Design review of the part shown in the three views and the two pictorial views. Dimensions are in mm from the part's minimum x, y and z. Round coordinates to 2 decimals unless told otherwise and drop trailing zeros. Loops run counter-clockwise (first coordinate to the right, second up) from the corner with the lowest first, then second, coordinate; pieces in that order, holes last. Notation, with made-up numbers: M -38.75,18.25 L 12.25,18.25 A23 cw 12.25,42.25 Z; hole C 79.5,75.5 d9. An arc over 180 degrees is marked long. Return JSON: item names as keys, results as strings. Group by question number.
Q1. Consider section B-B (z = 30). State the section outline as (x, y) points, and give its area (3 significant figures).
Q2. Draft analysis for pull direction X (two halves, no side actions). For the marked faces 1 and 2, state which applies: pulls with the +X half, pulls with the -X half, needs draft (parallel to the pull), parting line crosses it, or undercut.
Q3. Consider section C-C (x = 10). State the section outline as (y, z) points, and give its area (3 significant figures).
Q4. To check wall thickness, follow line 1 along X through (y, z) = (3.3, 30); line 2 along X through (y, z) = (2, 30); line 3 along X through (y, z) = (3.1, 28). State the ranges of each line that lie inside material, in increasing order.
Q5. Consider section D-D (z = 24). State the section outline as (x, y) points, and give its area (3 significant figures).
Q6. Consider section A-A (x = 30). State the section outline as (y, z) points, and give its area (3 significant figures).
Q7. Clearance check with flat-ended pins moving along their axes: pin 1 Ø3.5 at (x, z) = (30, 30) entering from +Y; pin 2 Ø1.7 at (y, z) = (2.5, 30) entering from +X; pin 3 Ø2 at (x, y) = (17.5, 2.5) entering from -Z; pin 4 Ø5 at (x, z) = (8, 29) entering from +Y. State where each tip first meets the part, or that it passes through.
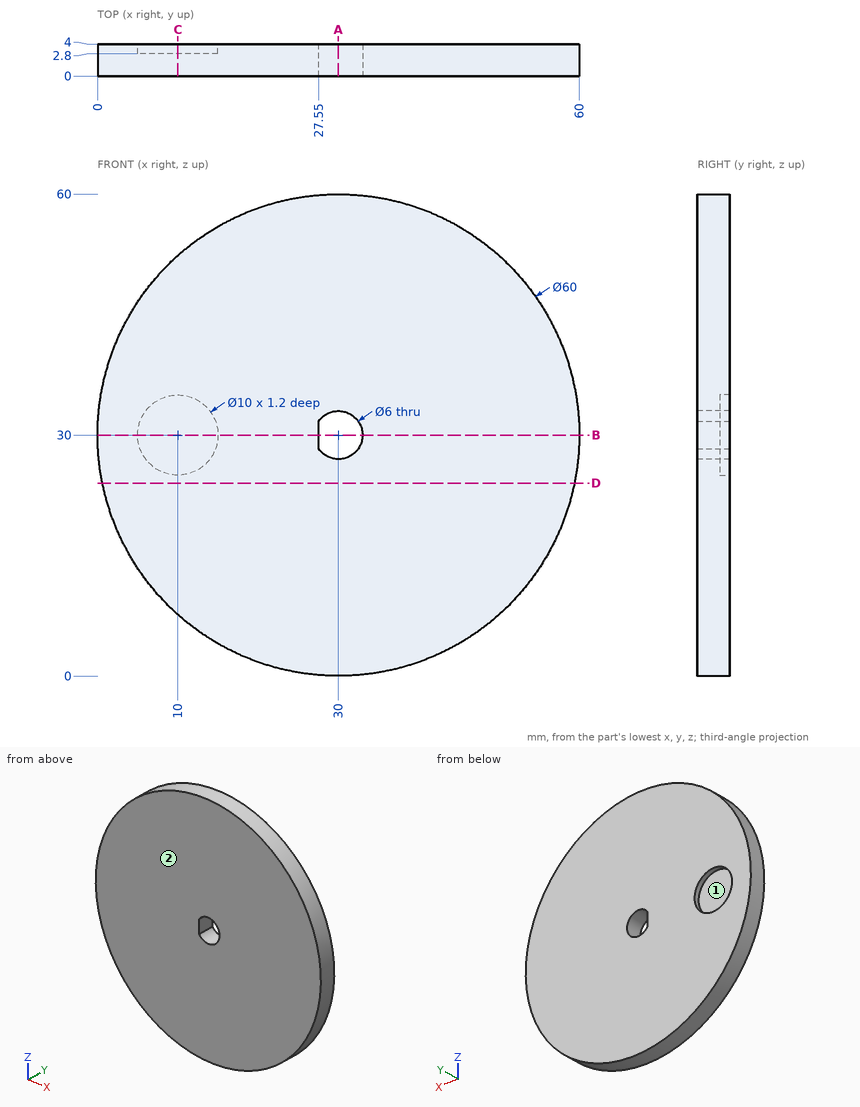
Values:
{
 "1": {"outline": "M 0,0 L 27.55,0 L 27.55,4 L 15,4 L 15,2.8 L 5,2.8 L 5,4 L 0,4 Z; M 33,0 L 60,0 L 60,4 L 33,4 Z", "area": "206 mm2"},
 "2": {"face 1": "undercut", "face 2": "needs draft"},
 "3": {"outline": "M 0,7.64 L 4,7.64 L 4,25 L 2.8,25 L 2.8,35 L 4,35 L 4,52.36 L 0,52.36 Z", "area": "167 mm2"},
 "4": {"line 1": "x = 0 to 5, 15 to 27.55, 33 to 60", "line 2": "x = 0 to 27.55, 33 to 60", "line 3": "x = 0.07 to 5.42, 14.58 to 27.76, 32.24 to 59.93"},
 "5": {"outline": "M 0.61,0 L 59.39,0 L 59.39,4 L 0.61,4 Z", "area": "235 mm2"},
 "6": {"outline": "M 0,0 L 4,0 L 4,27 L 0,27 Z; M 0,33 L 4,33 L 4,60 L 0,60 Z", "area": "216 mm2"},
 "7": {"pin 1": "passes through", "pin 2": "stops at x = 60", "pin 3": "stops at z = 2.29", "pin 4": "stops at y = 2.8"}
}
